Geometry check sheet. Reference: the model listing, model coordinates, mm. A direction names the side the tool comes from. Round coordinates to 2 decimals unless told otherwise and drop trailing zeros. Write each loop counter-clockwise with the first axis right and the second up, starting at its lowest first coordinate (ties: lowest second). Pieces come first, ordered by that corner, then holes. Notation, with made-up numbers: (2, -32.75) -> (9, -32.75) arc R9 ccw to (9, -25.75) -> close; hole circle Ø9 at (50.5, 33.5). An arc over 180 degrees is marked (long way). Use a Markdown table: item, result.
Autodesk Inventor part; units mm, degrees
ref_plane "YZ Plane" through (0, 0, 0) normal (1, 0, 0) x (0, 1, 0)
ref_plane "XZ Plane" through (0, 0, 0) normal (0, 1, 0) x (-1, 0, 0)
ref_plane "XY Plane" through (0, 0, 0) normal (0, 0, 1) x (1, 0, 0)
sketch "Náčrt1" plane through (0, 0, 0) normal (0, 0, 1) x (1, 0, 0)
  line L0 (0, 0) -> (-82.5, 0)
  line L1 (-82.5, 0) -> (-82.5, 11)
  line L2 (-82.5, 11) -> (-20.578, 11)
  line L3 (-20.578, 11) -> (-12, 15)
  line L4 (-12, 15) -> (0, 15)
  line L5 (0, 15) -> (0, 0)
  dimension "d2" = 22
  dimension "d3" = 30
  dimension "d4" = 12
  dimension "d5" = 25
  dimension "d6" = 82.5
revolve "Rotace1" add sketch "Náčrt1" angle 360 about axis through (0, 0, 0) along (-1, 0, 0)
hole "Díra1" at (0, 0, 0) direction (-1, 0, 0) diameter 22.38 depth 14 tip angle 118
hole "Díra2" at (0, 0, 0) direction (-1, 0, 0) diameter 19.2 depth 75 tip angle 118
hole "Díra3" at (-82.5, 0, 0) direction (1, 0, 0) diameter 8.92 depth 12 tip angle 118
chamfer "Zkosení1" distance 6 angle 30 1 edges at (-82.5, -11, 0) measured on face at (-41.2187, 10.8576, 1.7645)
sketch "Náčrt2" plane through (0, 0, 0) normal (1, 0, 0) x (0, 0, -1)
  circle A0 centre (16, 0) radius 2.6
  point P0 (0, 0)
  dimension "d40" = 16
  dimension "d41" = 5.2
extrude "Vysunutí1" cut sketch "Náčrt2" against normal blind 5
pattern_circular "Kruhové pole1" count 18 over 360 about axis through (-6, 0, 0) along (1, 0, 0) of "Vysunutí1"
chamfer "Zkosení2" distance 0.5 angle 45 1 edges at (0, 0, 11.19)
properties part number "Head01" material "ETG 100"
(1) Access from +Z, -Z, +X, -X, +Y, -Y to the whole of each face (thin tool, end or side, straight path). Record for faces 1 (the face through (-48.15, -2.38, -10.74)), 2 (the face through (-5, -12, -7)), 3 (the face through (-7.344, 10.924, 2.426)), 4 (the face through (-5, 0, -14)), 5 (the face through (-2.46, -4.62, 12.58)).
A:
| item | result |
|---|---|
| face 1 | -X |
| face 2 | +X, -Y |
| face 3 | +X |
| face 4 | -Z, +X |
| face 5 | +Z, +X |
(2) Section check C-C on x = -9. Record the cut outline in (y, z), plus the area to 3 significant figures.
A:
| item | result |
|---|---|
| outline | circle Ø30 at (0, 0); hole circle Ø22.38 at (0, 0) |
| area | 313 mm2 |
(3) Thickness scan on line 1 (Z direction, x = -7.5, y = 0); line 2 (Y direction, x = -56, z = 0). Record the ranges inside material, lowest first.
A:
| item | result |
|---|---|
| line 1 | z = -15 to -11.19, 11.19 to 15 |
| line 2 | y = -11 to -9.6, 9.6 to 11 |
(4) Section check B-B on x = -40.5. Record the cut outline in (y, z).
A:
| item | result |
|---|---|
| outline | circle Ø22 at (0, 0); hole circle Ø19.2 at (0, 0) |
(5) Gauge pin test, flat ends, axial feed: pin 1 Ø6 at (y, z) = (2.5, -7) entering from +X; pin 2 Ø1.1 at (y, z) = (-4.5, -14) entering from +X; pin 3 Ø15.5 at (y, z) = (0, 0) entering from +X; pin 4 Ø10 at (y, z) = (11.5, 3) entering from -X. Record the tip position at first contact, or that the pin passes through.
A:
| item | result |
|---|---|
| pin 1 | stops at x = -14.45 |
| pin 2 | stops at x = -5 |
| pin 3 | stops at x = -76.11 |
| pin 4 | stops at x = -82.5 |
(6) Section check A-A on y = 0. Record the cut outline in (x, z), plus the area to 3 significant figures.
A:
| item | result |
|---|---|
| outline | (-82.5, -7.54) -> (-76.5, -11) -> (-20.58, -11) -> (-12, -15) -> (-5, -15) -> (-5, -13.4) -> (0, -13.4) -> (0, -11.69) -> (-0.5, -11.19) -> (-14, -11.19) -> (-14.96, -9.6) -> (-75, -9.6) -> (-78.09, -4.46) -> (-82.5, -4.46) -> close; (-82.5, 4.46) -> (-78.09, 4.46) -> (-75, 9.6) -> (-14.96, 9.6) -> (-14, 11.19) -> (-0.5, 11.19) -> (0, 11.69) -> (0, 13.4) -> (-5, 13.4) -> (-5, 15) -> (-12, 15) -> (-20.58, 11) -> (-76.5, 11) -> (-82.5, 7.54) -> close |
| area | 339 mm2 |
